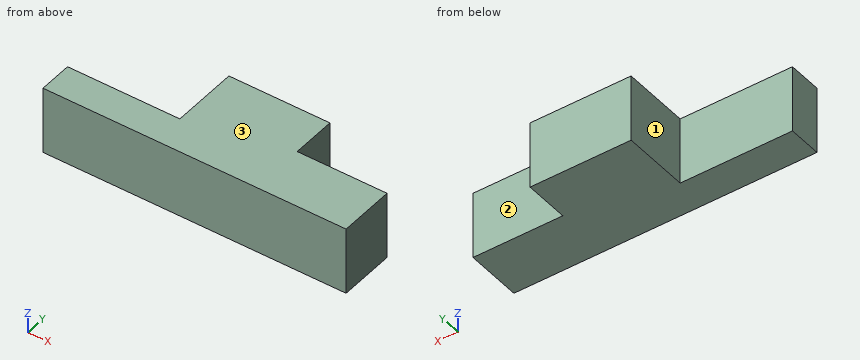
from build123d import *

# Parameters (mm, degrees)
SCHIZZO1_W                   = 50
SCHIZZO1_H                   = 30
ESTRUSIONE_ESTRUSIONE1_DEPTH = 15
SCHIZZO3_W                   = 45
SCHIZZO3_H                   = 15
ESTRUSIONE_ESTRUSIONE2_DEPTH = 15
SCHIZZO4_W                   = 45
SCHIZZO4_H                   = 30
ESTRUSIONE_ESTRUSIONE3_DEPTH = 15
SCHIZZO5_W                   = 40
SCHIZZO5_H                   = 30
ESTRUSIONE_ESTRUSIONE4_DEPTH = 25


with BuildPart() as part:
    # Schizzo1 → Estrusione-Estrusione1 (new body)
    with BuildSketch(Plane(origin=(0, 0, 0), x_dir=(1, 0, 0), z_dir=(0, 1, 0))):
        with Locations((-25, 0)):
            Rectangle(SCHIZZO1_W, SCHIZZO1_H)
    extrude(amount=ESTRUSIONE_ESTRUSIONE1_DEPTH)

    # Schizzo3 → Estrusione-Estrusione2 (add, symmetric)
    with BuildSketch(Plane.XY):
        with Locations((22.5, 7.5)):
            Rectangle(SCHIZZO3_W, SCHIZZO3_H)
    extrude(amount=ESTRUSIONE_ESTRUSIONE2_DEPTH, both=True)

    # Schizzo4 → Estrusione-Estrusione3 (add, symmetric)
    with BuildSketch(Plane.XY):
        with Locations((22.5, 30)):
            Rectangle(SCHIZZO4_W, SCHIZZO4_H)
    extrude(amount=ESTRUSIONE_ESTRUSIONE3_DEPTH, both=True)

    # Schizzo5 → Estrusione-Estrusione4 (add)
    with BuildSketch(Plane(origin=(0, 0, 0), x_dir=(1, 0, 0), z_dir=(0, 1, 0))):
        with Locations((65, 0)):
            Rectangle(SCHIZZO5_W, SCHIZZO5_H)
    extrude(amount=ESTRUSIONE_ESTRUSIONE4_DEPTH)


solid = part.part
Geometry: final body of the model. Coordinates: model frame, mm. Face numbers are marked on the shaded views. A direction names the side the tool comes from. Coordinates: 2 decimals unless noted, no trailing zeros. Loops run counter-clockwise (first coordinate to the right, second up) from the corner with the lowest first, then second, coordinate; pieces in that order, holes last. Notation, with made-up numbers: (32.5, 72.5) - (90.5, 72.5) arc R34 ccw to (90.5, 109.5) - close; hole circle Ø5 at (7, -32.75). An arc over 180 degrees is marked (long way). Put each result on its own line as item: value. Start each with the question number.
Q1. Cut plane A-A, the plane z = 3.5. Return loops of the section in (x, y), and give its area (4 significant figures).
Q2. Cut plane C-C, the plane x = 55. Return loops of the section in (y, z).
Q3. Pin query (flat end, axial travel): pin 1 Ø3 at (x, z) = (58, -1) entering from +Y; pin 2 Ø3 at (y, z) = (38.5, -9) entering from -X; pin 3 Ø6 at (y, z) = (31, 7) entering from +X. Return the tip coordinate at first contact, or that it passes through.
Q4. Line query: line 1 (Y direction, x = -34.5, z = 11.5); line 2 (X direction, y = 18, z = 1); line 3 (Y direction, x = 67.5, z = 13.75). Output: solid intervals per line, ascending.
Q5. Cut plane B-B, the plane y = 31.5. Return loops of the section in (x, z).
Q6. Set-up query: the marked faces 1, 2 and 3. Return all of +Z, -Z, +X, -X, +Y, -Y with unobstructed straight access to the full face (end or side cutting, diameter ignored); none if empty.
Filled sheet:
1. outline: (-50, 0) - (85, 0) - (85, 25) - (45, 25) - (45, 45) - (0, 45) - (0, 15) - (-50, 15) - close
1. area: 3,775 mm²
2. outline: (0, -15) - (25, -15) - (25, 15) - (0, 15) - close
3. pin 1: y = 25
3. pin 2: x = 0
3. pin 3: x = 45
4. line 1: 0 to 15
4. line 2: 0 to 85
4. line 3: 0 to 25
5. outline: (0, -15) - (45, -15) - (45, 15) - (0, 15) - close
6. face 1: +Z, -Z, -X, +Y
6. face 2: +Z, -Z, +X, +Y
6. face 3: +Z, +X, -X, +Y, -Y
